Check sheet for the modelled part. Datum: model origin and axes. Units: mm. Face numbers are marked on the shaded views. A direction names the side the tool comes from. Give positions to 0.01 mm unless a question says otherwise; leave off trailing zeros. Order: outer loops, then holes, each group sorted by start corner. A loop starts at its lowest first (then second) coordinate and runs counter-clockwise, first axis right, second up.
```python
from build123d import *

# Parameters (mm, degrees)
BOSS_EXTRUDE1_START     = 25
SKETCH1_W               = 3
SKETCH1_H               = 27
BOSS_EXTRUDE1_DEPTH     = 8
BOSS_EXTRUDE2_START     = 32.5
SKETCH2_W               = 3
SKETCH2_H               = 14
BOSS_EXTRUDE2_DEPTH     = 25.5
BOSS_EXTRUDE3_START     = 25
SKETCH3_W               = 8
SKETCH3_H               = 4.5
BOSS_EXTRUDE3_DEPTH     = 3
BOSS_EXTRUDE4_START     = 22
SKETCH4_W               = 3
SKETCH4_H               = 3.9
BOSS_EXTRUDE4_DEPTH     = 3
CUT_EXTRUDE1_DEPTH      = 65.845971347
CUT_EXTRUDE1_DEPTH_BACK = 65.845971347
SKETCH5_R               = 1.2
CUT_EXTRUDE2_DEPTH      = 65.845971347
CUT_EXTRUDE2_DEPTH_BACK = 65.845971347
SKETCH6_W               = 1.8
SKETCH6_H               = 1
CUT_EXTRUDE3_DEPTH      = 65.845971347
CUT_EXTRUDE3_DEPTH_BACK = 65.845971347


with BuildPart() as part:
    # Sketch1 → Boss-Extrude1 (new body)
    with BuildSketch(Plane.XY.offset(BOSS_EXTRUDE1_START)):
        with Locations((11.5, 6.5)):
            Rectangle(SKETCH1_W, SKETCH1_H)
    extrude(amount=BOSS_EXTRUDE1_DEPTH)

    # Sketch2 → Boss-Extrude2 (add)
    with BuildSketch(Plane.XY.offset(BOSS_EXTRUDE2_START)):
        with Locations((11.5, 0)):
            Rectangle(SKETCH2_W, SKETCH2_H)
    extrude(amount=BOSS_EXTRUDE2_DEPTH)

    # Sketch3 → Boss-Extrude3 (add)
    with BuildSketch(Plane.XY.offset(BOSS_EXTRUDE3_START)):
        with Locations((17, 17.725)):
            Rectangle(SKETCH3_W, SKETCH3_H)
    extrude(amount=BOSS_EXTRUDE3_DEPTH)

    # Sketch4 → Boss-Extrude4 (add)
    with BuildSketch(Plane.XY.offset(BOSS_EXTRUDE4_START)):
        with Locations((11.5, 17.725)):
            Rectangle(SKETCH4_W, SKETCH4_H)
    extrude(amount=BOSS_EXTRUDE4_DEPTH)

    # Sketch5 → Cut-Extrude1 (cut, two sides: drawn at the far end of the back side and taken through both)
    with BuildSketch(Plane.XY.offset(-CUT_EXTRUDE1_DEPTH_BACK)):
        with Locations((15, 17.725)):
            Circle(SKETCH5_R)
        with Locations((18.5, 17.725)):
            Circle(SKETCH5_R)
    extrude(amount=CUT_EXTRUDE1_DEPTH + CUT_EXTRUDE1_DEPTH_BACK, mode=Mode.SUBTRACT)

    # Sketch6 → Cut-Extrude2 (cut, two sides: drawn at the far end of the back side and taken through both)
    with BuildSketch(Plane(origin=(0, 0, 0), x_dir=(1, 0, 0), z_dir=(0, 1, 0)).offset(-CUT_EXTRUDE2_DEPTH_BACK)):
        with Locations((9.9, -29.5)):
            Rectangle(SKETCH6_W, SKETCH6_H)
        with Locations((9.9, -32)):
            Rectangle(SKETCH6_W, SKETCH6_H)
        with Locations((9.9, -34.5)):
            Rectangle(SKETCH6_W, SKETCH6_H)
        with Locations((9.9, -37)):
            Rectangle(SKETCH6_W, SKETCH6_H)
        with Locations((9.9, -39.5)):
            Rectangle(SKETCH6_W, SKETCH6_H)
        with Locations((9.9, -42)):
            Rectangle(SKETCH6_W, SKETCH6_H)
        with Locations((9.9, -44.5)):
            Rectangle(SKETCH6_W, SKETCH6_H)
        with Locations((9.9, -47)):
            Rectangle(SKETCH6_W, SKETCH6_H)
        with Locations((9.9, -49.5)):
            Rectangle(SKETCH6_W, SKETCH6_H)
        with Locations((9.9, -52)):
            Rectangle(SKETCH6_W, SKETCH6_H)
    extrude(amount=CUT_EXTRUDE2_DEPTH + CUT_EXTRUDE2_DEPTH_BACK, mode=Mode.SUBTRACT)

    # Sketch7 → Cut-Extrude3 (cut, two sides: drawn at the far end of the back side and taken through both)
    with BuildSketch(Plane(origin=(0, 0, 0), x_dir=(0, 0, -1), z_dir=(1, 0, 0)).offset(-CUT_EXTRUDE3_DEPTH_BACK)):
        Polygon((-55.3, -7.7), (-59, -7.7), (-59, -4), align=None)
        Polygon((-55.3, 7.7), (-59, 4), (-59, 7.7), align=None)
        Polygon((-28, 21), (-34, 21), (-34, 15), align=None)
    extrude(amount=CUT_EXTRUDE3_DEPTH + CUT_EXTRUDE3_DEPTH_BACK, mode=Mode.SUBTRACT)


solid = part.part
```
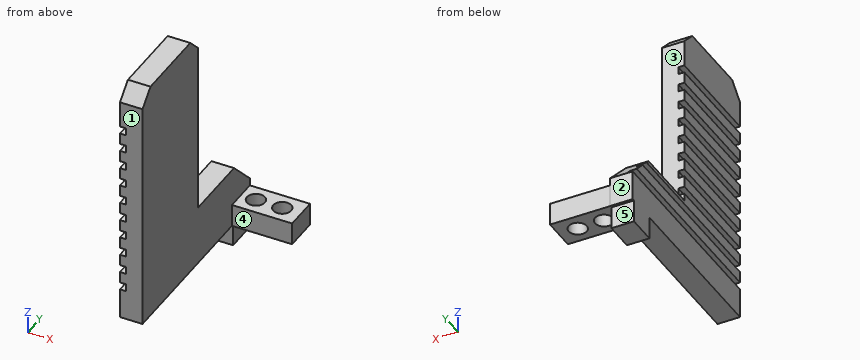
(1) Gauge pin test, flat ends, axial feed: pin 1 Ø4 at (y, z) = (5, 27.5) entering from +X; pin 2 Ø0.5 at (y, z) = (-1, 44.5) entering from -X; pin 3 Ø2.5 at (x, z) = (17.5, 27) entering from +Y (3 decimals). Record the tip position at first contact, or that the pin passes through.
Response values:
pin 1: stops at x = 13
pin 2: stops at x = 10.8
pin 3: stops at y = 19.975
(2) Cross-section at B-B on y = 17. Enter the section's corners in (x, z).
Response values:
outline: (10, 22) - (13, 22) - (13, 25) - (14.04, 25) - (14.04, 28) - (13, 28) - (13, 32) - (10.8, 32) - (10.8, 31.5) - (10, 31.5) - (10, 30) - (10.8, 30) - (10.8, 29) - (10, 29) - close; (15.96, 25) - (17.54, 25) - (17.54, 28) - (15.96, 28) - close; (19.46, 25) - (21, 25) - (21, 28) - (19.46, 28) - close
(3) Cross-section at C-C on z = 30.5. Enter the section's corners in (x, y), then the cut area to 3 significant figures.
Response values:
outline: (10, -7) - (13, -7) - (13, 18.5) - (10, 18.5) - close
area: 76.5 mm2
(4) Set-up check for the marked faces 1, 2, 3, 4 and 5: record each of +Z, -Z, +X, -X, +Y, -Y from which the full face is reachable in a straight line by a thin tool's end or side.
Response values:
face 1: +Z, -Z, +X, -X, -Y
face 2: +Z, -Z, +X, -X, +Y
face 3: +Z, +X, -X, +Y
face 4: +Z, -Z, +X, -Y
face 5: -Z, +X, -X, +Y
(5) Cross-section at D-D on x = 19. Enter the section's corners in (y, z) (3 decimals), then the cut area to 3 significant figures.
Response values:
outline: (15.475, 25) - (16.634, 25) - (16.634, 28) - (15.475, 28) - close; (18.816, 25) - (19.975, 25) - (19.975, 28) - (18.816, 28) - close
area: 6.95 mm2
(6) Material ranges on L1, parallel to Y at x = 18.5, z = 26.4 (3 decimals); L2, parallel to X at y = 1, z = 41; L3, parallel to Z at x = 11.75, y = 13, recorded low to high.
Response values:
L1: y = 15.475 to 16.525, 18.925 to 19.975
L2: x = 10 to 13
L3: z = 25 to 33
(7) Cross-section at A-A on x = 15. Enter the section's corners in (y, z) (3 decimals), then the cut area to 3 significant figures.
Response values:
outline: (15.475, 25) - (16.525, 25) - (16.525, 28) - (15.475, 28) - close; (18.925, 25) - (19.975, 25) - (19.975, 28) - (18.925, 28) - close
area: 6.30 mm2
